```python
from build123d import *

# Parameters (mm, degrees)
SKETCH1_R           = 2.54
BOSS_EXTRUDE1_DEPTH = 3.175
CHAMFER1_SIZE       = 31.75
FILLET1_R           = 6.35


with BuildPart() as part:
    # Sketch1 → Boss-Extrude1 (new body)
    with BuildSketch(Plane(origin=(0, 0, 0), x_dir=(1, 0, 0), z_dir=(0, 1, 0))):
        Polygon((25.4, 0), (0, 0), (0, -101.6), (-60.96, -101.6), (-60.96, -127), (25.4, -127), align=None)
        with Locations(Location((1.27, -114.3, 0), (0, 0, 270))):
            Circle(SKETCH1_R, mode=Mode.SUBTRACT)
        with Locations(Location((12.7, -12.7, 0), (0, 0, 270))):
            Circle(SKETCH1_R, mode=Mode.SUBTRACT)
        with Locations(Location((12.7, -38.1, 0), (0, 0, 270))):
            Circle(SKETCH1_R, mode=Mode.SUBTRACT)
        with Locations(Location((-24.13, -114.3, 0), (0, 0, 270))):
            Circle(SKETCH1_R, mode=Mode.SUBTRACT)
        with Locations(Location((-49.53, -114.3, 0), (0, 0, 270))):
            Circle(SKETCH1_R, mode=Mode.SUBTRACT)
    extrude(amount=BOSS_EXTRUDE1_DEPTH)

    # Chamfer1
    chamfer1_edges = [part.edges().sort_by_distance(p)[0] for p in [
        (0, 1.5875, 101.6),
    ]]
    chamfer(chamfer1_edges, length=CHAMFER1_SIZE)

    # Fillet1
    fillet1_edges = [part.edges().sort_by_distance(p)[0] for p in [
        (-60.96, 1.5875, 101.6),
        (0, 1.5875, 0),
        (25.4, 1.5875, 0),
        (25.4, 1.5875, 127),
        (-60.96, 1.5875, 127),
        (-31.75, 1.5875, 101.6),
        (0, 1.5875, 69.85),
    ]]
    fillet(fillet1_edges, radius=FILLET1_R)


solid = part.part
```
Input: part model. Units: mm. Frame: model coordinates. A direction names the side the tool comes from. Give positions to 0.01 mm unless a question says otherwise; leave off trailing zeros. Write each loop counter-clockwise with the first axis right and the second up, starting at its lowest first coordinate (ties: lowest second). Pieces come first, ordered by that corner, then holes. Notation, with made-up numbers: (35.25, -3) - (80.25, -3) arc R36 cw to (80.25, 35) - close; hole circle Ø10 at (-7.75, 84). An arc over 180 degrees is marked (long way). Write item = value, one per line. Start each with the question number.
1. First-contact query: pin 1 Ø1.5 at (x, y) = (2, 1.5) entering from -Z; pin 2 Ø1.6 at (x, y) = (-47, 1.5) entering from -Z; pin 3 Ø1.6 at (y, z) = (1, 35) entering from -X; pin 4 Ø3 at (x, z) = (-24.13, 114.3) entering from -Y. Flat tips, straight axial feed; report the tip coordinate or a pass-through.
2. Mould query, pull axis Z, two halves, no side actions, for faces 1 (the cylindrical face through (1.382, 1.565, 111.762)), 2 (the cylindrical face through (1.81, 1.61, 1.91)), 3 (the flat face through (0, 2, 36)), 4 (the cylindrical face through (-59.15, 1.61, 125.09)). Classes: released by +Z, released by -Z, zero draft, split by the parting line, or undercut.
3. Section query D-D, the plane y = 1.7. Output: boundary loops of the cut face in (x, z), then the cut area to 3 significant figures.
4. Section query B-B, the plane z = 114.3. Output: boundary loops of the cut face in (x, y) (3 decimals), then the cut area to 3 significant figures.
5. Ray query, L1, parallel to X at y = 2.15, z = 114.3; L2, parallel to X at y = 0.8, z = 38.1; L3, parallel to Z at x = 11, y = 3.05. Return the intervals inside material, ascending.
6. Section query A-A, the plane x = 12.7. Output: boundary loops of the cut face in (y, z) (3 decimals).
7. Section query C-C, the plane x = -24.13. Output: boundary loops of the cut face in (y, z) (3 decimals), then the cut area to 3 significant figures.
8. Access query for faces 5 (the flat face through (13, 2, 0)), 6 (the flat face through (-44, 2, 101.6)). Directions: +Z, -Z, +X, -X, +Y, -Y. A direction counts if a zero-diameter tool reaches every point of the face in a straight line with its end or side. Return the directions, or none.
Check sheet entries:
q1.pin_1 = 1.12
q1.pin_2 = 101.6
q1.pin_3 = 0
q1.pin_4 = through
q2.face_1 = undercut
q2.face_2 = released by -Z
q2.face_3 = zero draft
q2.face_4 = released by +Z
q3.outline = (-60.96, 107.95) arc R6.35 ccw to (-54.61, 101.6) - (-34.38, 101.6) arc R6.35 cw to (-29.89, 99.74) - (-1.86, 71.71) arc R6.35 cw to (0, 67.22) - (0, 6.35) arc R6.35 ccw to (6.35, 0) - (19.05, 0) arc R6.35 ccw to (25.4, 6.35) - (25.4, 120.65) arc R6.35 ccw to (19.05, 127) - (-54.61, 127) arc R6.35 ccw to (-60.96, 120.65) - close; hole circle Ø5.08 at (-49.53, 114.3); hole circle Ø5.08 at (-24.13, 114.3); hole circle Ø5.08 at (1.27, 114.3); hole circle Ø5.08 at (12.7, 12.7); hole circle Ø5.08 at (12.7, 38.1)
q3.area = 5,140 mm2
q4.outline = (-60.96, 0) - (-52.07, 0) - (-52.07, 3.175) - (-60.96, 3.175) - close; (-46.99, 0) - (-26.67, 0) - (-26.67, 3.175) - (-46.99, 3.175) - close; (-21.59, 0) - (-1.27, 0) - (-1.27, 3.175) - (-21.59, 3.175) - close; (3.81, 0) - (25.4, 0) - (25.4, 3.175) - (3.81, 3.175) - close
q4.area = 226 mm2
q5.L1 = -60.96 to -52.07, -46.99 to -26.67, -21.59 to -1.27, 3.81 to 25.4
q5.L2 = 0 to 10.16, 15.24 to 25.4
q5.L3 = 0 to 10.81, 14.59 to 36.21, 39.99 to 127
q6.outline = (0, 0) - (3.175, 0) - (3.175, 10.16) - (0, 10.16) - close; (0, 15.24) - (3.175, 15.24) - (3.175, 35.56) - (0, 35.56) - close; (0, 40.64) - (3.175, 40.64) - (3.175, 127) - (0, 127) - close
q7.outline = (0, 93.98) - (3.175, 93.98) - (3.175, 111.76) - (0, 111.76) - close; (0, 116.84) - (3.175, 116.84) - (3.175, 127) - (0, 127) - close
q7.area = 88.7 mm2
q8.face_5 = -Z, +X, -X, +Y, -Y
q8.face_6 = -Z, -X, +Y, -Y
